Autodesk Inventor part; units mm, degrees
ref_plane "Start Plane" through (0, 0, 17.9828) normal (0, 0, 1) x (1, 0, 0)
ref_plane "End Plane" through (0, 0, 382.0172) normal (0, 0, 1) x (1, 0, 0)
ref_plane "Work Plane4" through (536.0982, -972, -478.1154) normal (-0.7071, 0, -0.7071) x (-0.7071, 0, 0.7071)
ref_plane "Start Plane" through (0, 0, 17.9828) normal (0, 0, 1) x (1, 0, 0)
ref_plane "End Plane" through (0, 0, 382.0172) normal (0, 0, 1) x (1, 0, 0)
sketch "Sketch" plane through (0, 0, 0) normal (0, 0, 1) x (1, 0, 0)
  line L0 (-40, -28) -> (-40, 28)
  line L1 (-28, 40) -> (28, 40)
  line L2 (40, 28) -> (40, -28)
  line L3 (28, -40) -> (-28, -40)
  arc A0 (-40, -28) -> (-28, -40) centre (-28, -28) ccw
  arc A1 (-28, 40) -> (-40, 28) centre (-28, 28) ccw
  arc A2 (40, 28) -> (28, 40) centre (28, 28) ccw
  arc A3 (28, -40) -> (40, -28) centre (28, -28) ccw
  arc A4 (-28, 32) -> (-32, 28) centre (-28, 28) ccw
  line L4 (-28, 32) -> (28, 32)
  arc A5 (32, 28) -> (28, 32) centre (28, 28) ccw
  line L5 (32, 28) -> (32, -28)
  arc A6 (28, -32) -> (32, -28) centre (28, -28) ccw
  line L6 (28, -32) -> (-28, -32)
  arc A7 (-32, -28) -> (-28, -32) centre (-28, -28) ccw
  line L7 (-32, -28) -> (-32, 28)
  line L8 (0, 59.4794) -> (0, -59.4794) construction
  line L9 (-59.4794, 0) -> (59.4794, 0) construction
  dimension "d7" = 12
  dimension "d10" = 80
  dimension "d11" = 80
  dimension "d12" = 8
  dimension "d15" = 40
  dimension "d16" = 40
extrude "Body" add sketch "Sketch" along normal up to surface (364.0345 mm away) from surface at 17.9828
sketch "Sketch3" plane through (0, 0, 0) normal (0, 0, 1) x (1, 0, 0)
  line L0 (0, 0) -> (10, 0)
ref_plane "Work Plane3" through (0, 0, 0) normal (0, -1, 0) x (1, 0, 0)
ref_plane "Work Plane4" through (536.0982, -972, -478.1154) normal (-0.7071, 0, -0.7071) x (-0.7071, 0, 0.7071)
split "Split1" plane through (536.0982, -972, -478.1154) removes the side toward (-0.7071, 0, -0.7071)
ref_plane "Work Plane5" through (-171.0086, 28, 171.0086) normal (-0.7071, 0, 0.7071) x (0.7071, 0, 0.7071)
split "Split2" plane through (-171.0086, 28, 171.0086) removes the side toward (-0.7071, 0, 0.7071)
sketch "Sketch4" plane through (0, 0, 0) normal (0, -1, 0) x (1, 0, 0)
  line L0 (-2, 17.9828) -> (12, 17.9828)
  line L1 (-2, 382.0172) -> (12, 382.0172)
  dimension "d18" = 364.0345
equation "\"d7\" = G_IR"
equation "\"d10\" = G_H"
equation "\"d11\" = G_W"
equation "\"d12\" = G_T"
equation "\"d15\" = 0.5 * d10"
equation "\"d16\" = 0.5 * d11"
equation "\"d3\" = G_L"
equation "\"G_W\" = 80"
equation "\"G_H\" = 80"
equation "\"G_T\" = 8"
equation "\"G_IR\" = 12"
equation "\"G_L\" = d18"
equation "\"G_OFFSET_START\" = -17.98276"
equation "\"G_OFFSET_END\" = -17.98276"
equation "\"d13\" = -G_OFFSET_START"
equation "\"d14\" = G_OFFSET_END + B_L"
equation "\"B_L\" = 400"
properties part number "ISO 12633-2 - 80x80x8 - 364.03" material "Steel, Mild"
The model under review builds one solid part; all positions refer to its coordinate system, in mm. A direction names the side the tool comes from. Round coordinates to 2 decimals unless told otherwise and drop trailing zeros. Write each loop counter-clockwise with the first axis right and the second up, starting at its lowest first coordinate (ties: lowest second). Pieces come first, ordered by that corner, then holes. Notation, with made-up numbers: M 48.5,-15 L 99.5,-15 A16 ccw 99.5,-11 Z; hole C -26.75,80.5 d6. An arc over 180 degrees is marked long. Use CSV: the item, a comma, the result in double quotes. Start each with the question number.
(1) We need section B-B, the plane x = -9. State the section outline as (y, z) points.
(2) We need section C-C, the plane y = -6. State the section outline as (x, z) points.
(3) For line 1 along X through (y, z) = (15, 257.5); line 2 along X through (y, z) = (3.5, 315), list the stretches that pass through material, from the lowest coordinate up.
(4) The part is to be moulded in two halves that separate along Y. For faces 1 (the face through (0, -32, 198)), 2 (the face through (40, 0, 197)), 3 (the face through (36.58, -36.39, 197.45)), say which applies: +Y half, -Y half, draft (parallel to the pull), parting line (faces both ways), or undercut.
(5) We need section D-D, the plane z = 318. State the section outline as (x, y) points, then the cut area to 3 significant figures.
(6) Tool access review of faces 4 (the face through (0, 40, 198)), 5 (the face through (-32, 0, 198)): name each direction out of +Z, -Z, +X, -X, +Y, -Y from which nothing blocks a thin tool from reaching the whole face with its end or side.
(7) We need section A-A, the plane z = 118. State the section outline as (x, y) points, then the cut area to 3 significant figures.
Findings:
1,outline,"M -40,66.98 L -32,66.98 L -32,333.02 L -40,333.02 Z; M 32,66.98 L 40,66.98 L 40,333.02 L 32,333.02 Z"
2,outline,"M -40,97.98 L -32,89.98 L -32,310.02 L -40,302.02 Z; M 32,25.98 L 40,17.98 L 40,382.02 L 32,374.02 Z"
3,line 1,"-40 to -32, 32 to 40"
3,line 2,"32 to 40"
4,face 1,"undercut"
4,face 2,"draft"
4,face 3,"-Y half"
5,outline,"M -24.02,-40 L 28,-40 A12 ccw 40,-28 L 40,28 A12 ccw 28,40 L -24.02,40 L -24.02,32 L 28,32 A4 cw 32,28 L 32,-28 A4 cw 28,-32 L -24.02,-32 Z"
5,area,"1,480 mm^2"
6,face 4,"+Z, -Z, +X, -X, +Y"
6,face 5,"+Z, -Z"
7,outline,"M -40,-28 A12 ccw -28,-40 L 28,-40 A12 ccw 40,-28 L 40,28 A12 ccw 28,40 L -28,40 A12 ccw -40,28 Z; hole M -32,-28 A4 ccw -28,-32 L 28,-32 A4 ccw 32,-28 L 32,28 A4 ccw 28,32 L -28,32 A4 ccw -32,28 Z"
7,area,"2,190 mm^2"
